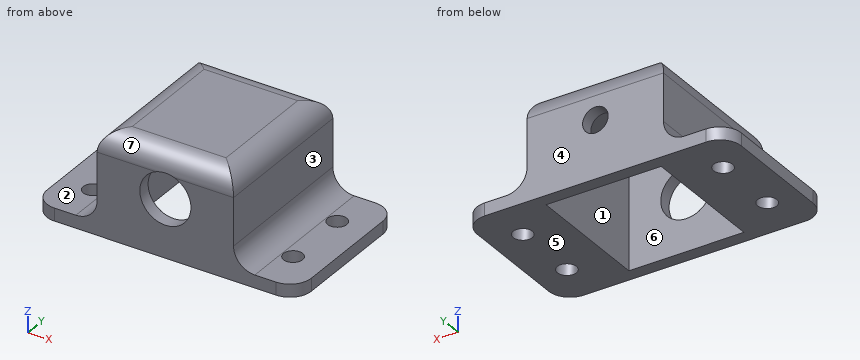
```python
from build123d import *

# Parameters (mm, degrees)
F0_W        = 32
F0_H        = 21.1520095187
F0_R        = 6
F1_DEPTH    = 30
F2_T        = -2.5
F3_DEPTH    = 3
F4_W        = 32
F4_H        = 21.1520095187
F4_R        = 3
F5_DEPTH    = 3
F6_R        = 2.25
F7_DEPTH    = 3
F8_T1_DEPTH = 36
F8_T3_DEPTH = 61
F8_T5_DEPTH = 57
F8_T7_DEPTH = 28


# Not quite as in the source:
# - a fillet or chamfer that OpenCascade refuses, or shapes differently, is made with other operations: its cross-section is extruded or revolved along the edge and cut away or added
# - a feature names something its author has since deleted; it is built from what else it names


with BuildPart() as f1:
    # F0 (on Front) → F1 (new body)
    with BuildSketch(Plane.XZ):
        Rectangle(F0_W, F0_H)
        Circle(F0_R, mode=Mode.SUBTRACT)
        Circle(F0_R)
    extrude(amount=-F1_DEPTH)

    # F2
    f2_openings = [f1.faces().sort_by_distance(p)[0] for p in [
        (0, 0, 0),
        (0, 30, 0),
        (0, 15, -10.576005),
    ]]
    offset(amount=F2_T, openings=f2_openings)

    # F0 (on Front) → F3 (join)
    with BuildSketch(Plane.XZ):
        Rectangle(F0_W, F0_H)
        Circle(F0_R, mode=Mode.SUBTRACT)
    extrude(amount=F3_DEPTH)

    # F4 (on face) → F5 (join)
    with BuildSketch(Plane(origin=(0, 30, 0), x_dir=(-1, 0, 0), z_dir=(0, 1, 0))):
        Rectangle(F4_W, F4_H)
        Circle(F4_R, mode=Mode.SUBTRACT)
    extrude(amount=F5_DEPTH)

    # F6 (on face) → F7 (join)
    with BuildSketch(Plane(origin=(0, 0, -10.5760047594), x_dir=(1, 0, 0), z_dir=(0, 0, -1))):
        Polygon((-16, 3), (-16, 0), (-13.5, 0), (13.5, 0), (16, 0), (16, 3), align=None)
        Polygon((-16, -33), (-16, 0), (-16, 3), (-31, 3), (-31, -33), align=None)
        with Locations((-23.5, -23)):
            Circle(F6_R, mode=Mode.SUBTRACT)
        with Locations((-23.5, -7)):
            Circle(F6_R, mode=Mode.SUBTRACT)
        Polygon((-13.5, 0), (-16, 0), (-16, -33), (16, -33), (16, 0), (13.5, 0), (13.5, -30), (-13.5, -30), align=None)
        Polygon((31, 3), (16, 3), (16, 0), (16, -33), (31, -33), align=None)
        with Locations((23.5, -23)):
            Circle(F6_R, mode=Mode.SUBTRACT)
        with Locations((23.5, -7)):
            Circle(F6_R, mode=Mode.SUBTRACT)
    extrude(amount=F7_DEPTH)

    # F8: fillet of radius 5 on 10 edges, made by hand

    # F8_s2 → F8_t1 (join)
    with BuildSketch(Plane.XZ.offset(-33)):
        with BuildLine():
            ThreePointArc((-16, -5.5760047594), (-17.4644660941, -9.1115386653), (-21, -10.5760047594))
            Line((-21, -10.5760047594), (-16, -10.5760047594))
            Line((-16, -10.5760047594), (-16, -5.5760047594))
        make_face()
        with BuildLine():
            ThreePointArc((16, -5.5760047594), (17.4644660941, -9.1115386653), (21, -10.5760047594))
            Line((21, -10.5760047594), (16, -10.5760047594))
            Line((16, -10.5760047594), (16, -5.5760047594))
        make_face()
    extrude(amount=F8_T1_DEPTH)

    # F8_s4 → F8_t3 (cut)
    with BuildSketch(Plane.XZ.offset(-45.5)):
        with BuildLine():
            ThreePointArc((-11, 10.5760047594), (-14.5355339059, 9.1115386653), (-16, 5.5760047594))
            Line((-16, 5.5760047594), (-16, 10.5760047594))
            Line((-16, 10.5760047594), (-11, 10.5760047594))
        make_face()
        with BuildLine():
            ThreePointArc((16, 5.5760047594), (14.5355339059, 9.1115386653), (11, 10.5760047594))
            Line((11, 10.5760047594), (16, 10.5760047594))
            Line((16, 10.5760047594), (16, 5.5760047594))
        make_face()
    extrude(amount=F8_T3_DEPTH, mode=Mode.SUBTRACT)

    # F8_s6 → F8_t5 (cut)
    with BuildSketch(Plane.YZ.offset(-28.5)):
        with BuildLine():
            ThreePointArc((-3, 5.5760047594), (-1.5355339059, 9.1115386653), (2, 10.5760047594))
            Line((2, 10.5760047594), (-3, 10.5760047594))
            Line((-3, 10.5760047594), (-3, 5.5760047594))
        make_face()
        with BuildLine():
            ThreePointArc((28, 10.5760047594), (31.5355339059, 9.1115386653), (33, 5.5760047594))
            Line((33, 5.5760047594), (33, 10.5760047594))
            Line((33, 10.5760047594), (28, 10.5760047594))
        make_face()
    extrude(amount=F8_T5_DEPTH, mode=Mode.SUBTRACT)

    # F8_s8 → F8_t7 (cut)
    with BuildSketch(Plane.XY.offset(-26.0760047594)):
        with BuildLine():
            ThreePointArc((26, -3), (29.5355339059, -1.5355339059), (31, 2))
            Line((31, 2), (31, -3))
            Line((31, -3), (26, -3))
        make_face()
        with BuildLine():
            ThreePointArc((26, 33), (29.5355339059, 31.5355339059), (31, 28))
            Line((31, 28), (31, 33))
            Line((31, 33), (26, 33))
        make_face()
        with BuildLine():
            ThreePointArc((-26, -3), (-29.5355339059, -1.5355339059), (-31, 2))
            Line((-31, 2), (-31, -3))
            Line((-31, -3), (-26, -3))
        make_face()
        with BuildLine():
            ThreePointArc((-26, 33), (-29.5355339059, 31.5355339059), (-31, 28))
            Line((-31, 28), (-31, 33))
            Line((-31, 33), (-26, 33))
        make_face()
    extrude(amount=F8_T7_DEPTH, mode=Mode.SUBTRACT)


solid = f1.part
```
Geometry: final body of the model. Coordinates: model frame, mm. Face numbers are marked on the shaded views. A direction names the side the tool comes from. Give positions to 0.01 mm unless a question says otherwise; leave off trailing zeros. Loops run counter-clockwise (first coordinate to the right, second up) from the corner with the lowest first, then second, coordinate; pieces in that order, holes last. Notation, with made-up numbers: (12.25, 13) -> (68.25, 13) arc R20 ccw to (68.25, 29) -> close; hole circle Ø8 at (60, 30.25). An arc over 180 degrees is marked (long way). Use one line per item in the form item = value.
Item 1: Line query: probe 1 along X at (y, z) = (7, -12.2); probe 2 along Y at (x, z) = (23.5, -11.25); probe 3 along X at (y, z) = (9, -1). Output: solid intervals per line, ascending.
A:
probe_1 = -31 to -25.75, -21.25 to -13.5, 13.5 to 21.25, 25.75 to 31
probe_2 = -3 to 4.75, 9.25 to 20.75, 25.25 to 33
probe_3 = -16 to -13.5, 13.5 to 16
Item 2: Section query D-D on z = -8.25. Output: boundary loops of the cut face in (x, y), and give its area (3 significant figures).
A:
outline = (-16.78, -3) -> (16.78, -3) -> (16.78, 33) -> (-16.78, 33) -> close; hole (-13.5, 0) -> (13.5, 0) -> (13.5, 30) -> (-13.5, 30) -> close
area = 398 mm^2
Item 3: Section query B-B on x = 23.5. Output: boundary loops of the cut face in (y, z).
A:
outline = (-3, -13.58) -> (4.75, -13.58) -> (4.75, -10.58) -> (-3, -10.58) -> close; (9.25, -13.58) -> (20.75, -13.58) -> (20.75, -10.58) -> (9.25, -10.58) -> close; (25.25, -13.58) -> (33, -13.58) -> (33, -10.58) -> (25.25, -10.58) -> close
Item 4: Section query C-C on y = 7. Output: boundary loops of the cut face in (x, z), and give its area (3 significant figures).
A:
outline = (-31, -13.58) -> (-25.75, -13.58) -> (-25.75, -10.58) -> (-31, -10.58) -> close; (-21.25, -13.58) -> (-13.5, -13.58) -> (-13.5, 8.08) -> (13.5, 8.08) -> (13.5, -13.58) -> (21.25, -13.58) -> (21.25, -10.58) -> (21, -10.58) arc R5 cw to (16, -5.58) -> (16, 5.58) arc R5 ccw to (11, 10.58) -> (-11, 10.58) arc R5 ccw to (-16, 5.58) -> (-16, -5.58) arc R5 cw to (-21, -10.58) -> (-21.25, -10.58) -> close; (25.75, -13.58) -> (31, -13.58) -> (31, -10.58) -> (25.75, -10.58) -> close
area = 251 mm^2
Item 5: Pin query (flat end, axial travel): P1, Ø3, axis at x = 27.5, y = 19, coming from the +Z side; P2, Ø3.5, axis at y = 9, z = 1.5, coming from the -X side; P3, Ø12.5, axis at y = 14.5, z = 2, coming from the +X side. Return the tip coordinate at first contact, or that it passes through.
A:
P1 = -10.58
P2 = -16
P3 = 16
Item 6: Draft query along Y for the marked faces 4, 5, 6 and 7. Return one class per face: pulls with the +Y half, pulls with the -Y half, needs draft (parallel to the pull), parting line crosses it, or undercut.
A:
face_4 = pulls with the +Y half
face_5 = needs draft
face_6 = undercut
face_7 = pulls with the -Y half
Item 7: Section query A-A on z = 0. Output: boundary loops of the cut face in (x, y).
A:
outline = (-16, -3) -> (-6, -3) -> (-6, 0) -> (-13.5, 0) -> (-13.5, 30) -> (-3, 30) -> (-3, 33) -> (-16, 33) -> close; (3, 30) -> (13.5, 30) -> (13.5, 0) -> (6, 0) -> (6, -3) -> (16, -3) -> (16, 33) -> (3, 33) -> close
Item 8: Access query for the marked faces 1, 2 and 3. Directions: +Z, -Z, +X, -X, +Y, -Y. A direction counts if a zero-diameter tool reaches every point of the face in a straight line with its end or side. Return the directions, or none.
A:
face_1 = -Z
face_2 = +Z, -X, +Y, -Y
face_3 = +Z, +X, +Y, -Y
